```python
from build123d import *

# Parameters (mm, degrees)
F0_W     = 11.7856
F0_H     = 29.972
F1_DEPTH = 1.9685
F2_R     = 0.762
F3_R     = 0.5334
F4_DEPTH = 3.81


with BuildPart() as f1:
    # F0 (on Top) → F1 (new body, symmetric)
    with BuildSketch(Plane.XY):
        Rectangle(F0_W, F0_H)
    extrude(amount=F1_DEPTH, both=True)

    # F2
    f2_edges = [f1.edges().sort_by_distance(p)[0] for p in [
        (-5.8928, 0, 1.9685),
        (-5.8928, 0, -1.9685),
        (5.8928, 0, -1.9685),
        (5.8928, 0, 1.9685),
    ]]
    fillet(f2_edges, radius=F2_R)

    # F3 (on face) → F4 (join)
    with BuildSketch(Plane(origin=(0, 14.986, 0), x_dir=(-1, 0, 0), z_dir=(0, 1, 0))):
        with Locations((-3.3528, -1.4351)):
            Circle(F3_R)
        with Locations((-0.8128, -1.4351)):
            Circle(F3_R)
    extrude(amount=F4_DEPTH)


solid = f1.part
```
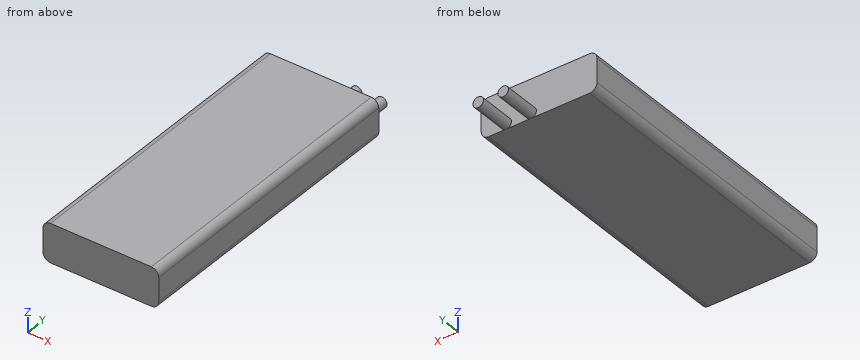
Input: part model. Units: mm. Frame: model coordinates. Round coordinates to 2 decimals unless told otherwise and drop trailing zeros. Loops run counter-clockwise (first coordinate to the right, second up) from the corner with the lowest first, then second, coordinate; pieces in that order, holes last. Notation, with made-up numbers: (19, 1) - (71, 1) arc R13 cw to (71, 20) - close; hole circle Ø4 at (27.5, 85). An arc over 180 degrees is marked (long way). One line per item, written item: value. Start each with the question number.
(1) Section A-A, the plane z = 0.1. Return loops of the section in (x, y).
(2) Section B-B, the plane x = -0.75. Return loops of the section in (y, z).
(3) Ray query, line 1 (Y direction, x = -2.5, z = 0.85); line 2 (Z direction, x = 5.75, y = -5.5); line 3 (Z direction, x = 5.5, y = 9). Return the intervals inside material, ascending. Write a range as [from, to].
(4) Contact query for a flat-ended pin moving along its axis: P1, Ø1.2, axis at x = 2, z = -0.5, coming from the +Y side. Output: stop coordinate, or through.
Results below:
1. outline: (-5.89, -14.99) - (5.89, -14.99) - (5.89, 14.99) - (-5.89, 14.99) - close
2. outline: (-14.99, -1.97) - (14.99, -1.97) - (14.99, 1.97) - (-14.99, 1.97) - close
3. line 1: [-14.99, 14.99]
3. line 2: [-1.65, 1.65]
3. line 3: [-1.87, 1.87]
4. P1: y = 14.99
